from build123d import *

# Parameters (mm, degrees)
F0_R      = 26
F3_DEPTH  = 20
F4_DEPTH  = 5
F2_R      = 18
F5_DEPTH  = 30
F6_R      = 17
F8_DEPTH  = 5
F7_R      = 9.5
F9_DEPTH  = 20
F10_R     = 10
F11_DEPTH = 25


with BuildPart() as f3:
    # F0 (on Top) → F3 (new body)
    with BuildSketch(Plane.XY):
        Circle(F0_R)
    extrude(amount=F3_DEPTH)

    # F1 (on Top) → F4 (join)
    with BuildSketch(Plane.XY):
        Polygon((100, 18), (0, 26), (0, -26), (100, -18), align=None)
    extrude(amount=F4_DEPTH)

    # F2 (on Top) → F5 (join)
    with BuildSketch(Plane.XY):
        with Locations((100, 0)):
            Circle(F2_R)
    extrude(amount=F5_DEPTH)

    # F6 (on face) → F8 (join)
    with BuildSketch(Plane.XY.offset(20)):
        Circle(F6_R)
    extrude(amount=F8_DEPTH)

    # F7 (on face) → F9 (join)
    with BuildSketch(Plane.XY.offset(30)):
        with Locations((100, 0)):
            Circle(F7_R)
    extrude(amount=F9_DEPTH)

    # F10 (on face) → F11 (cut, through all)
    with BuildSketch(Plane.XY.offset(25)):
        Circle(F10_R)
    extrude(amount=-F11_DEPTH, mode=Mode.SUBTRACT)


solid = f3.part
Geometry: final body of the model. Coordinates: model frame, mm. A direction names the side the tool comes from. Give positions to 0.01 mm unless a question says otherwise; leave off trailing zeros. Order: outer loops, then holes, each group sorted by start corner. A loop starts at its lowest first (then second) coordinate and runs counter-clockwise, first axis right, second up. Notation, with made-up numbers: (4, 12) -> (56, 12) arc R17 ccw to (56, 37) -> close; hole circle Ø8 at (83.5, 79.25). An arc over 180 degrees is marked (long way). Answer as a JSON object with one key per item and string values.
Q1. Section C-C (z = 23.5). Output: boundary loops of the cut face in (x, y).
Entries:
{"outline": "circle Ø34 at (0, 0); circle Ø36 at (100, 0); hole circle Ø20 at (0, 0)"}
Q2. Access query for faces 1 (the cylindrical face through (-25.975, 1.143, 9.86)), 2 (the flat face through (45, 0, 0)), 3 (the flat face through (7.3, -7.3, 25)). Directions: +Z, -Z, +X, -X, +Y, -Y. A direction counts if a zero-diameter tool reaches every point of the face in a straight line with its end or side. Return the directions, or none.
Entries:
{"face 1": "+Z", "face 2": "-Z, +X, -X, +Y, -Y", "face 3": "+Z, -X, +Y, -Y"}
Q3. Section D-D (x = 20). Output: boundary loops of the cut face in (y, z).
Entries:
{"outline": "(-24.4, 0) -> (24.4, 0) -> (24.4, 5) -> (16.61, 5) -> (16.61, 20) -> (-16.61, 20) -> (-16.61, 5) -> (-24.4, 5) -> close"}
Q4. First-contact query: pin 1 (1 mm diameter, centred on y = 14.5, z = 12, fed in from -X); pin 2 (3 mm diameter, centred on y = -5, z = 22.5, fed in from +X); pin 3 (5 mm diameter, centred on y = 9, z = 41, fed in from -X). Flat tips, straight axial feed; report the tip coordinate or a pass-through.
Entries:
{"pin 1": "stops at x = -21.91", "pin 2": "stops at x = 117.66", "pin 3": "stops at x = 93.07"}
Q5. Draft query along Y for faces 4 (the flat face through (100, 0, 50)), 5 (the cylindrical face through (109.061, 2.854, 39.86)), 6 (the cylindrical face through (-2.17, -9.76, 12.68)), 7 (the flat face through (51.4, -21.89, 2.46)). Return one class per face: released by +Y, released by -Y, zero draft, split by the parting line, or undercut.
Entries:
{"face 4": "zero draft", "face 5": "split by the parting line", "face 6": "undercut", "face 7": "released by -Y"}
Q6. Section A-A (x = 0). Output: boundary loops of the cut face in (y, z), plus the area to 3 significant figures.
Entries:
{"outline": "(-26, 0) -> (-10, 0) -> (-10, 25) -> (-17, 25) -> (-17, 20) -> (-26, 20) -> close; (10, 0) -> (26, 0) -> (26, 20) -> (17, 20) -> (17, 25) -> (10, 25) -> close", "area": "710 mm^2"}
Q7. Section B-B (y = 0). Output: boundary loops of the cut face in (x, z).
Entries:
{"outline": "(-26, 0) -> (-10, 0) -> (-10, 25) -> (-17, 25) -> (-17, 20) -> (-26, 20) -> close; (10, 0) -> (118, 0) -> (118, 30) -> (109.5, 30) -> (109.5, 50) -> (90.5, 50) -> (90.5, 30) -> (82, 30) -> (82, 5) -> (26, 5) -> (26, 20) -> (17, 20) -> (17, 25) -> (10, 25) -> close"}
Q8. Material intervals for probe 1 along Y at (x, z) = (0, 7.5); probe 2 along Z at (x, y) = (30.5, 13); probe 3 along Z at (x, y) = (-0.5, 22), sorted ascending.
Entries:
{"probe 1": "y = -26 to -10, 10 to 26", "probe 2": "z = 0 to 5", "probe 3": "z = 0 to 20"}
